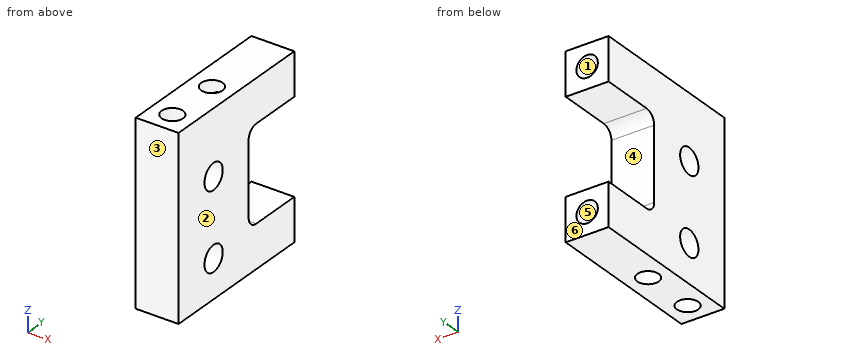
from build123d import *

# Parameters (mm, degrees)
ESQUISSE1_W           = 42
ESQUISSE1_H           = 38
EXTRUSION1_DEPTH      = 10
ESQUISSE2_R           = 2.5
EXTRUSION3_DEPTH      = 58.515215378
EXTRUSION4_REACH      = 59.515
EXTRUSION4_END_RADIUS = 2.5
ESQUISSE4_R           = 2.5
EXTRUSION5_DEPTH      = 58.515215378
ESQUISSE6_R           = 3
EXTRUSION6_DEPTH      = 58.515215378


with BuildPart() as part:
    # Esquisse1 → Extrusion1 (new body)
    with BuildSketch(Plane(origin=(0, 0, 0), x_dir=(0, 0, -1), z_dir=(1, 0, 0))):
        with Locations((21, 19)):
            Rectangle(ESQUISSE1_W, ESQUISSE1_H)
    extrude(amount=EXTRUSION1_DEPTH)

    # Esquisse2 → Extrusion3 (cut, through all)
    with BuildSketch(Plane.XY):
        with Locations((5, 5)):
            Circle(ESQUISSE2_R)
        with Locations((5, 18)):
            Circle(ESQUISSE2_R)
    extrude(amount=-EXTRUSION3_DEPTH, mode=Mode.SUBTRACT)

    # Extrusion4: up to this cylinder (the profile starts outside it)
    extrusion4_end = Plane(origin=(5, 18, -21), z_dir=(0, 0, 1)) * Cylinder(EXTRUSION4_END_RADIUS, 157.03, mode=Mode.PRIVATE)
    # Esquisse4 → Extrusion4 (cut, up to the surface)
    with BuildSketch(Plane(origin=(0, 38, 0), x_dir=(1, 0, 0), z_dir=(0, 1, 0)), mode=Mode.PRIVATE) as extrusion4_sk1:
        with Locations(Location((5, 5, 0), (0, 0, 270))):
            Circle(ESQUISSE4_R)
    extrusion4_tool1 = extrude(extrusion4_sk1.sketch, amount=-EXTRUSION4_REACH, mode=Mode.PRIVATE) - extrusion4_end
    add(extrusion4_tool1.solids().sort_by_distance((5, 38, -5))[0], mode=Mode.SUBTRACT)
    # Esquisse4 → Extrusion4 (cut, up to the surface)
    with BuildSketch(Plane(origin=(0, 38, 0), x_dir=(1, 0, 0), z_dir=(0, 1, 0)), mode=Mode.PRIVATE) as extrusion4_sk2:
        with Locations(Location((5, 37, 0), (0, 0, 270))):
            Circle(ESQUISSE4_R)
    extrusion4_tool2 = extrude(extrusion4_sk2.sketch, amount=-EXTRUSION4_REACH, mode=Mode.PRIVATE) - extrusion4_end
    add(extrusion4_tool2.solids().sort_by_distance((5, 38, -37))[0], mode=Mode.SUBTRACT)

    # Esquisse5 → Extrusion5 (cut, through all)
    with BuildSketch(Plane.ZY):
        with BuildLine():
            Line((-32, 40.062963014), (-10, 40.062963014))
            Line((-10, 40.062963014), (-10, 25.5))
            ThreePointArc((-10, 25.5), (-10.732233047, 23.732233047), (-12.5, 23))
            Line((-12.5, 23), (-29.5, 23))
            ThreePointArc((-29.5, 23), (-31.267766953, 23.732233047), (-32, 25.5))
            Line((-32, 25.5), (-32, 40.062963014))
        make_face()
    extrude(amount=-EXTRUSION5_DEPTH, mode=Mode.SUBTRACT)

    # Esquisse6 → Extrusion6 (cut, through all)
    with BuildSketch(Plane.ZY):
        with Locations((-33, 11.5)):
            Circle(ESQUISSE6_R)
        with Locations((-15, 11.5)):
            Circle(ESQUISSE6_R)
    extrude(amount=-EXTRUSION6_DEPTH, mode=Mode.SUBTRACT)


solid = part.part
Could you check a few things on this model? Use its own coordinates, in mm. Face numbers are marked on the shaded views. A direction names the side the tool comes from. Coordinates: 2 decimals unless noted, no trailing zeros. Order: outer loops, then holes, each group sorted by start corner. A loop starts at its lowest first (then second) coordinate and runs counter-clockwise, first axis right, second up. Notation, with made-up numbers: (45.25, 4) -> (51.25, 4) arc R18 ccw to (51.25, 10) -> close; hole circle Ø3 at (68, 79.5). An arc over 180 degrees is marked (long way). One line per item, written item: value. Start each with the question number.
1) Imagine slicing it at C-C on y = 26. List the corners of the cut face in (x, z) for me.
2) Imagine slicing it at A-A on x = 5. List the corners of the cut face in (y, z) for me.
3) We'd pull the mould along X, two halves only. Please class the marked faces 1, 2 and 3: +X half, -X half, draft (parallel to the pull), parting line (faces both ways), or undercut.
4) Imagine slicing it at D-D on y = 5. List the corners of the cut face in (x, z) for me, plus the area to 3 significant figures.
5) If I drill on L1, parallel to Y at x = 5, z = -8.5; L2, parallel to Z at x = 5, y = 27; L3, parallel to X at y = 18, z = -12, over which ranges is the centre line in solid material (lowest first)? Write a range as [from, to].
6) Imagine slicing it at B-B on z = -15. List the corners of the cut face in (x, y) for me.
7) Which directions (+Z, -Z, +X, -X, +Y, -Y) give clear straight access to the entire face, cutting with the end or side of a thin tool? Please do the marked faces 4, 5 and 6.
8) I'm going to push a flat-ended pin straight in: pin 1 (7 mm diameter, centred on y = 11.5, z = -33, fed in from -X). Where does the tip first touch, or does it pass through?
Answer list:
1. outline: (0, -42) -> (10, -42) -> (10, -32) -> (0, -32) -> close; (0, -10) -> (10, -10) -> (10, 0) -> (0, 0) -> close; hole circle Ø5 at (5, -37); hole circle Ø5 at (5, -5)
2. outline: (0, -42) -> (2.5, -42) -> (2.5, 0) -> (0, 0) -> close; (7.5, -42) -> (15.5, -42) -> (15.5, 0) -> (7.5, 0) -> close; (20.5, -42) -> (38, -42) -> (38, -39.5) -> (20.5, -39.5) -> close; (20.5, -34.5) -> (38, -34.5) -> (38, -32) -> (25.5, -32) arc R2.5 cw to (23, -29.5) -> (23, -12.5) arc R2.5 cw to (25.5, -10) -> (38, -10) -> (38, -7.5) -> (20.5, -7.5) -> close; (20.5, -2.5) -> (38, -2.5) -> (38, 0) -> (20.5, 0) -> close; hole circle Ø6 at (11.5, -33); hole circle Ø6 at (11.5, -15)
3. face 1: undercut
3. face 2: +X half
3. face 3: draft
4. outline: (0, -42) -> (2.5, -42) -> (2.5, 0) -> (0, 0) -> close; (7.5, -42) -> (10, -42) -> (10, 0) -> (7.5, 0) -> close
4. area: 210 mm2
5. L1: y = [0, 2.5], [7.5, 15.5], [20.5, 38]
5. L2: z = [-42, -39.5], [-34.5, -32], [-10, -7.5], [-2.5, 0]
5. L3: x = [0, 2.5], [7.5, 10]
6. outline: (0, 0) -> (10, 0) -> (10, 8.5) -> (0, 8.5) -> close; (0, 14.5) -> (10, 14.5) -> (10, 23) -> (0, 23) -> close; hole circle Ø5 at (5, 5); hole circle Ø5 at (5, 18)
7. face 4: +X, -X, +Y
7. face 5: +Y
7. face 6: +Z, -Z, +X, -X, +Y
8. pin 1: stops at x = 0
